Job drawing, mm, ordinate dimensions from the low corner. One solid piece. A direction names the side the tool comes from. Give positions to 0.01 mm unless a question says otherwise; leave off trailing zeros. Write each loop counter-clockwise with the first axis right and the second up, starting at its lowest first coordinate (ties: lowest second). Pieces come first, ordered by that corner, then holes. Notation, with made-up numbers: (35, 72.25) - (50, 72.25) arc R20 ccw to (50, 110.25) - close; hole circle Ø4 at (-22, -35.5). An arc over 180 degrees is marked (long way). Answer in a Markdown table with one row per item. Add a question column.
1. Band-saw the part on B-B on x = 4.5. State how many separate pieces and enclosed holes the cut face has, plus the area to 3 significant figures.
2. Band-saw the part on C-C on x = 9.5. Write the cut outline in (y, z), plus the area to 3 significant figures.
3. Band-saw the part on A-A on y = 5. Write the cut outline in (x, z).
4. Pull direction Z, two halves, no side cores. Call the marked faces 1, 2 and 3: released by +Z, released by -Z, zero draft, split by the parting line, or undercut.
5. Band-saw the part on D-D on y = 15. Write the cut outline in (x, z).
6. Drop flat-ended pins along their axis: pin 1 Ø4.5 at (x, y) = (3, 16.5) entering from -Z; pin 2 Ø2.5 at (y, z) = (14, 13) entering from -X; pin 3 Ø4 at (y, z) = (15, 15) entering from +X. Give the stop position or say it passes through.
7. Probe line 1 along X through (y, z) = (4, 11); line 2 along X through (y, z) = (4, 7); line 3 along Z through (x, y) = (3.75, 15). List the from-to ranges inside material, lowest first.
8. Which spindle directions (+Z, -Z, +X, -X, +Y, -Y) get a long thin tool onto all of the face, cutting with end or side? Do the marked faces 4, 5, 6 and 7. Say none if no direction does.
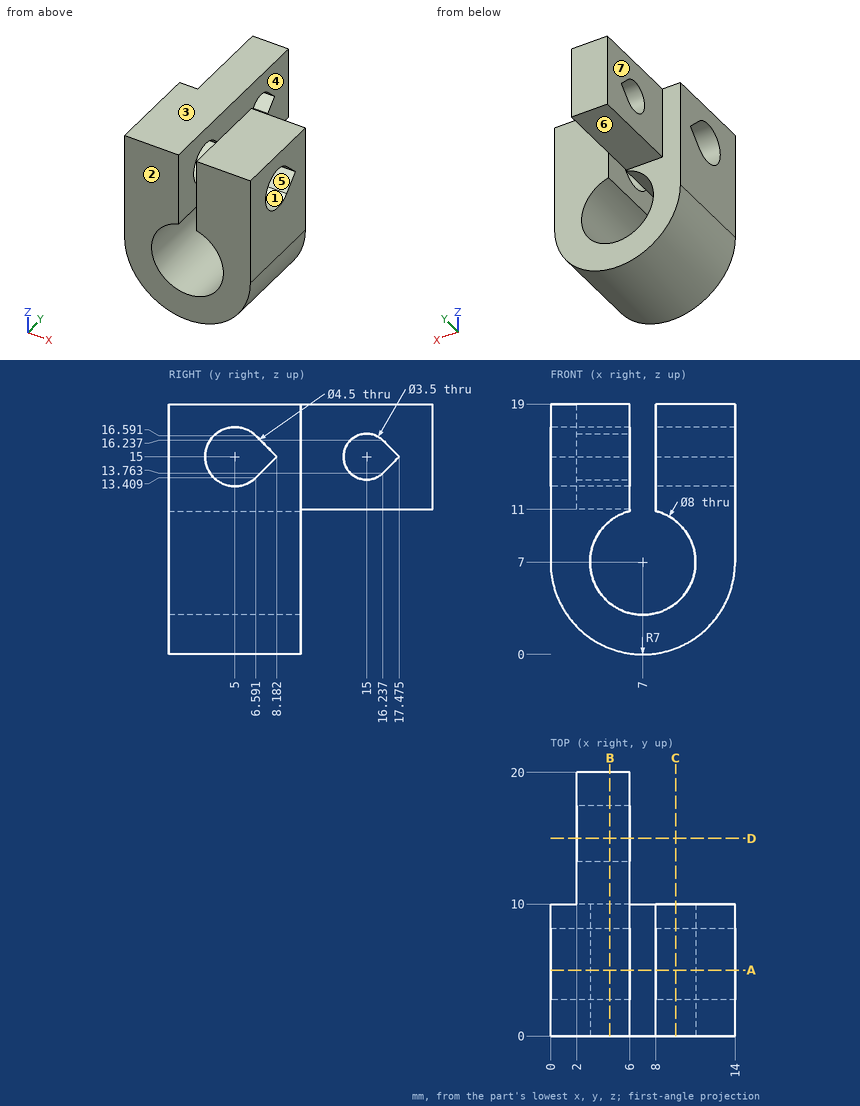
Values:
| question | item | result |
|---|---|---|
| 1 | separate pieces | 2 |
| 1 | enclosed holes | 2 |
| 1 | area | 176 mm² |
| 2 | outline | (0, 0.46) - (10, 0.46) - (10, 3.88) - (0, 3.88) - close; (0, 10.12) - (10, 10.12) - (10, 19) - (0, 19) - close; hole (6.59, 13.41) - (8.18, 15) - (6.59, 16.59) arc R2.25 ccw (long way) to start |
| 2 | area | 106 mm² |
| 3 | outline | (0, 7) arc R7 ccw to (14, 7) - (14, 12.75) - (8, 12.75) - (8, 10.87) arc R4 cw (long way) to (6, 10.87) - (6, 12.75) - (0, 12.75) - close; (0, 17.25) - (6, 17.25) - (6, 19) - (0, 19) - close; (8, 17.25) - (14, 17.25) - (14, 19) - (8, 19) - close |
| 4 | face 1 | undercut |
| 4 | face 2 | zero draft |
| 4 | face 3 | released by +Z |
| 5 | outline | (2, 11) - (6, 11) - (6, 13.25) - (2, 13.25) - close; (2, 16.75) - (6, 16.75) - (6, 19) - (2, 19) - close |
| 6 | pin 1 | stops at z = 11 |
| 6 | pin 2 | stops at x = 2 |
| 6 | pin 3 | stops at x = 6 |
| 7 | line 1 | x = 0 to 6, 8 to 14 |
| 7 | line 2 | x = 0 to 3, 11 to 14 |
| 7 | line 3 | z = 11 to 13.25, 16.75 to 19 |
| 8 | face 4 | +Z, +Y, -Y |
| 8 | face 5 | +X, -X |
| 8 | face 6 | -Z, +X, -X, +Y |
| 8 | face 7 | +Z, -Z, -X, +Y |
